from build123d import *

# Parameters (mm, degrees)
SKETCH1_R           = 44
BOSS_EXTRUDE1_DEPTH = 15
BOSS_EXTRUDE2_DEPTH = 5
SKETCH5_R           = 40
CUT_EXTRUDE1_DEPTH  = 20
CUT_EXTRUDE2_DEPTH  = 10
SKETCH7_R           = 3
CUT_EXTRUDE3_DEPTH  = 3
FILLET4_R           = 1


with BuildPart() as part:
    # Sketch1 → Boss-Extrude1 (new body)
    with BuildSketch(Plane(origin=(0, 0, 0), x_dir=(1, 0, 0), z_dir=(0, 1, 0))):
        with Locations(Location((0, 0, 0), (0, 0, 270))):
            Circle(SKETCH1_R)
    extrude(amount=BOSS_EXTRUDE1_DEPTH)

    # Sketch2 → Boss-Extrude2 (add)
    with BuildSketch(Plane(origin=(0, 15, 0), x_dir=(1, 0, 0), z_dir=(0, 1, 0))):
        with BuildLine():
            Line((15.246488352, -37.736382881), (15.845858901, -39.219877048))
            ThreePointArc((15.845858901, -39.219877048), (0, 42.3), (-15.845858901, -39.219877048))
            Line((-15.845858901, -39.219877048), (-15.246488352, -37.736382881))
            ThreePointArc((-15.246488352, -37.736382881), (0, 40.7), (15.246488352, -37.736382881))
        make_face()
    extrude(amount=BOSS_EXTRUDE2_DEPTH)

    # Sketch5 → Cut-Extrude1 (cut)
    with BuildSketch(Plane(origin=(0, 5.890466531, 0.803245436), x_dir=(-1, 0, 0), z_dir=(0, -0.990830168044299, -0.13511320473331362))):
        with Locations(Location((0, 0, 0), (0, 0, 270))):
            Circle(SKETCH5_R)
    extrude(amount=CUT_EXTRUDE1_DEPTH, mode=Mode.SUBTRACT)

    # Sketch6 → Cut-Extrude2 (cut)
    with BuildSketch(Plane(origin=(0, 5.890466531, 0.803245436), x_dir=(1, 0, 0), z_dir=(0, -0.990830168044299, -0.13511320473331365))):
        with BuildLine():
            ThreePointArc((-11.581105416, -33.107376853), (0, -38.033026978), (11.581105416, -33.107376853))
            ThreePointArc((11.581105416, -33.107376853), (11.503519007, -28.998721657), (7.39486381, -29.076308066))
            ThreePointArc((7.39486381, -29.076308066), (0, -32.221475176), (-7.39486381, -29.076308066))
            ThreePointArc((-7.39486381, -29.076308066), (-11.503519007, -28.998721657), (-11.581105416, -33.107376853))
        make_face()
    extrude(amount=-CUT_EXTRUDE2_DEPTH, mode=Mode.SUBTRACT)

    # Sketch7 → Cut-Extrude3 (cut)
    with BuildSketch(Plane(origin=(0, 6.082528488, -0.605208909), x_dir=(1, 0, 0), z_dir=(0, 0.990830168044299, 0.13511320473331365))):
        with Locations(Location((14.370787869, -14.421489162, 0), (0, 0, 270))):
            Circle(SKETCH7_R)
        with Locations(Location((-14.370787869, -14.421489162, 0), (0, 0, 90))):
            Circle(SKETCH7_R)
    extrude(amount=CUT_EXTRUDE3_DEPTH, mode=Mode.SUBTRACT)

    # Fillet4
    # the kernel refuses this fillet: 1 mm, written as the material it adds along each edge
    with BuildSketch(Plane(origin=(0, 5.890466531, 0.803245436), x_dir=(0, -0.13511320473331362, 0.9908301680442989), z_dir=(1, 0, 0))) as fillet4_piece_1_section:
        with BuildLine():
            CenterArc((40 - FILLET4_R, FILLET4_R), FILLET4_R, 270, 90)
            Line((40 - FILLET4_R, 0), (40, 0))
            Line((40, 0), (40, FILLET4_R))
        make_face()
    fillet4_piece_1 = revolve(axis=Axis((0, 5.890466531, 0.803245436), (0, -0.990830168044299, -0.13511320473331362)), mode=Mode.PRIVATE)
    fillet4_piece_1 = split(fillet4_piece_1, bisect_by=Plane(origin=(0, 0, -38.603422622), z_dir=(0, 1, 0)), keep=Keep.TOP, mode=Mode.PRIVATE)
    add(fillet4_piece_1)

    # Sketch9 → Revolve4 (revolve)
    with BuildSketch(Plane(origin=(0, 0, 0), x_dir=(1, 0, 0), z_dir=(0, 0.13511320473331362, -0.990830168044299)), mode=Mode.PRIVATE) as revolve4_sk:
        with BuildLine():
            Line((0, 4.055018992), (0, -5.944981008))
            Line((0, -5.944981008), (4.472135955, -5.944981008))
            ThreePointArc((4.472135955, -5.944981008), (5.477225575, 0.504508735), (0, 4.055018992))
        make_face()
    revolve(revolve4_sk.sketch.rotate(Axis((0, -4.017835149, -0.547886611), (0, 0.9908301680442989, 0.1351132047333136)), 90), axis=Axis((0, -4.017835149, -0.547886611), (0, 0.9908301680442989, 0.1351132047333136)))


solid = part.part
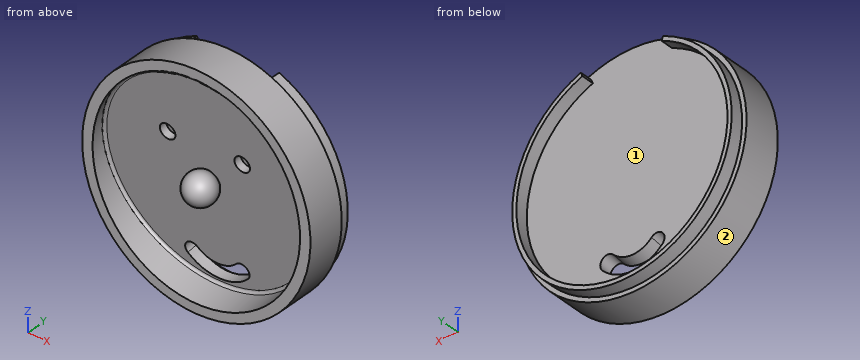
Geometry: final body of the model. Coordinates: model frame, mm. Face numbers are marked on the shaded views. Round coordinates to 2 decimals unless told otherwise and drop trailing zeros. Loops run counter-clockwise (first coordinate to the right, second up) from the corner with the lowest first, then second, coordinate; pieces in that order, holes last.
Q1. Section B-B on y = 2.5. State how many separate pieces and enclosed holes the cut face has, plus the area to 3 significant figures.
Q2. Pull-direction query (Z, two-part tool) for the marked faces 1 and 2; classes: released by +Z, released by -Z, zero draft, split by the parting line, or undercut.
Q3. Section A-A on x = 0. Return loops of the section in (y, z).
Q4. Section C-C on y = -2.5. Return loops of the section in (x, z), plus the area to 3 significant figures.
Q5. Material intervals for L1, parallel to X at y = 17.15, z = 0; L2, parallel to Y at x = -37.5, z = 18.5; L3, parallel to Z at x = -20.5, y = 1, sorted ascending.
Q6. Pin query (flat end, axial travel): P1, Ø4, axis at x = 18, z = -29.5, coming from the -Y side; P2, Ø1, axis at y = 1, z = 31, coming from the +X side; P3, Ø6, axis at x = 30, y = 11.5, coming from the +Z side. Return the tip coordinate at first contact, or that it passes through.
Evaluation:
1. separate pieces: 2
1. enclosed holes: 1
1. area: 1,780 mm2
2. face 1: undercut
2. face 2: split by the parting line
3. outline: (0, -44) - (15, -44) - (15, -42.3) - (20, -42.3) - (20, -40.7) - (15, -40.7) - (15, -36.34) - (11.03, -36.88) - (11.16, -37.84) arc R1 cw to (10.3, -38.97) - (0, -40.37) - close; (0, 40.24) arc R1 cw to (0.62, 39.45) - (5.29, 5.23) arc R6 ccw (long way) to (6.49, -3.63) - (10.24, -31.12) - (15, -30.47) - (15, 44) - (0, 44) - close
4. outline: circle Ø8.1 at (0, 0.26)
4. area: 51.5 mm2
5. L1: x = -42.3 to -40.7, 40.7 to 42.3
5. L2: y = 0 to 20
5. L3: z = -38.93 to -34.53, 34.46 to 38.93
6. P1: stops at y = 9.75
6. P2: stops at x = 31.71
6. P3: stops at z = 34.74
